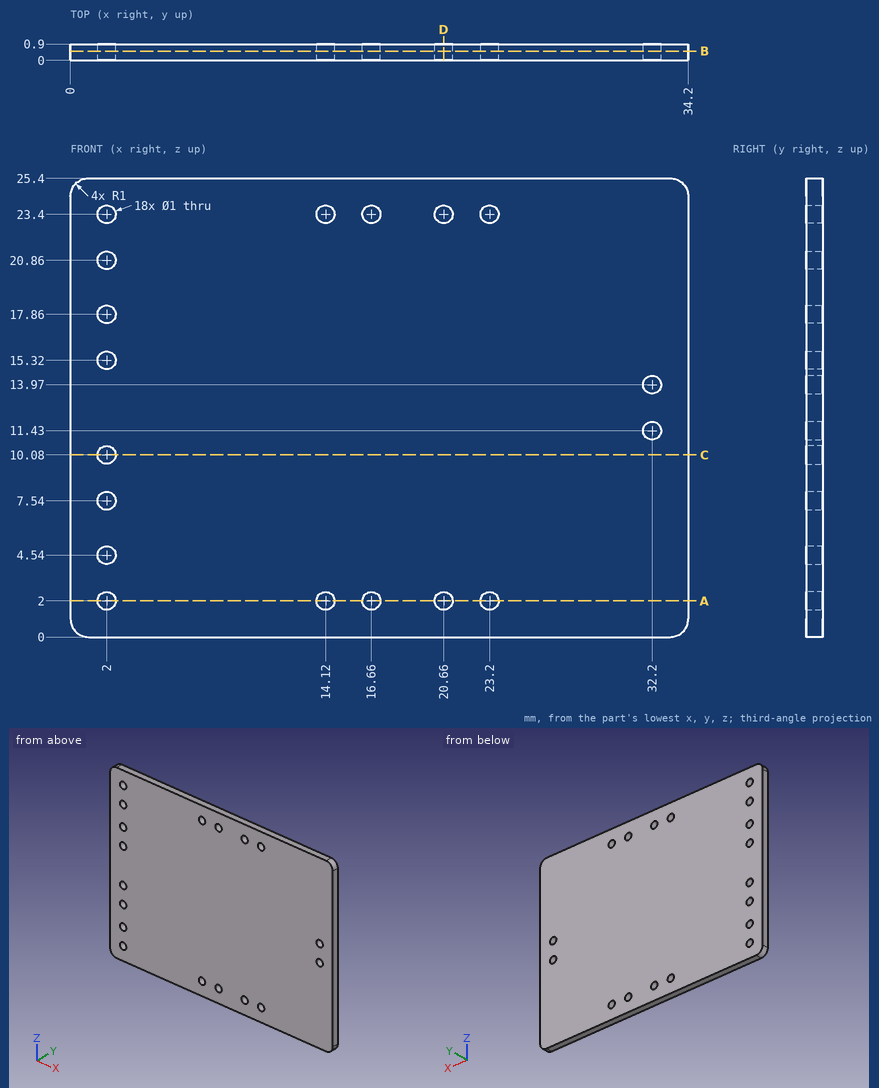
Job drawing, mm, ordinate dimensions from the low corner. One solid piece. Round coordinates to 2 decimals unless told otherwise and drop trailing zeros. Loops run counter-clockwise (first coordinate to the right, second up) from the corner with the lowest first, then second, coordinate; pieces in that order, holes last. Notation, with made-up numbers: (22, 63) -> (35, 63) arc R33 ccw to (35, 91) -> close; hole circle Ø10 at (76.5, -8.75). An arc over 180 degrees is marked (long way). Use a Markdown table: item, result.
1) Cut at C-C, the plane z = 10.08. List the corners of the cut face in (x, y).
The answers:
| item | result |
|---|---|
| outline | (0, 0) -> (1.5, 0) -> (1.5, 0.9) -> (0, 0.9) -> close; (2.5, 0) -> (34.2, 0) -> (34.2, 0.9) -> (2.5, 0.9) -> close |
2) Cut at B-B, the plane y = 0.5. State how many separate pieces and enclosed holes the cut face has, and give its area (3 significant figures).
The answers:
| item | result |
|---|---|
| separate pieces | 1 |
| enclosed holes | 18 |
| area | 854 mm2 |
3) Probe line 1 (X direction, y = 0.45, z = 23.4); line 2 (X direction, y = 0.7, z = 11.5); line 3 (X direction, y = 0.6, z = 20.86). List the from-to ranges inside material, lowest first. Write a range as [from, to].
The answers:
| item | result |
|---|---|
| line 1 | x = [0, 1.5], [2.5, 13.62], [14.62, 16.16], [17.16, 20.16], [21.16, 22.7], [23.7, 34.2] |
| line 2 | x = [0, 31.7], [32.7, 34.2] |
| line 3 | x = [0, 1.5], [2.5, 34.2] |
4) Cut at D-D, the plane x = 20.66. List the corners of the cut face in (y, z).
The answers:
| item | result |
|---|---|
| outline | (0, 0) -> (0.9, 0) -> (0.9, 1.5) -> (0, 1.5) -> close; (0, 2.5) -> (0.9, 2.5) -> (0.9, 22.9) -> (0, 22.9) -> close; (0, 23.9) -> (0.9, 23.9) -> (0.9, 25.4) -> (0, 25.4) -> close |
5) Cut at A-A, the plane z = 2. List the corners of the cut face in (x, y), and give its area (3 significant figures).
The answers:
| item | result |
|---|---|
| outline | (0, 0) -> (1.5, 0) -> (1.5, 0.9) -> (0, 0.9) -> close; (2.5, 0) -> (13.62, 0) -> (13.62, 0.9) -> (2.5, 0.9) -> close; (14.62, 0) -> (16.16, 0) -> (16.16, 0.9) -> (14.62, 0.9) -> close; (17.16, 0) -> (20.16, 0) -> (20.16, 0.9) -> (17.16, 0.9) -> close; (21.16, 0) -> (22.7, 0) -> (22.7, 0.9) -> (21.16, 0.9) -> close; (23.7, 0) -> (34.2, 0) -> (34.2, 0.9) -> (23.7, 0.9) -> close |
| area | 26.3 mm2 |
